Input: part model. Units: mm. Frame: model coordinates. Coordinates: 2 decimals unless noted, no trailing zeros. Write each loop counter-clockwise with the first axis right and the second up, starting at its lowest first coordinate (ties: lowest second). Pieces come first, ordered by that corner, then holes. Notation, with made-up numbers: (41, 85) - (45, 85) arc R4 cw to (45, 89) - close; hole circle Ø5 at (-20.5, 73.5). An arc over 180 degrees is marked (long way). Use CSV: the item, a comma, the result in double quotes.
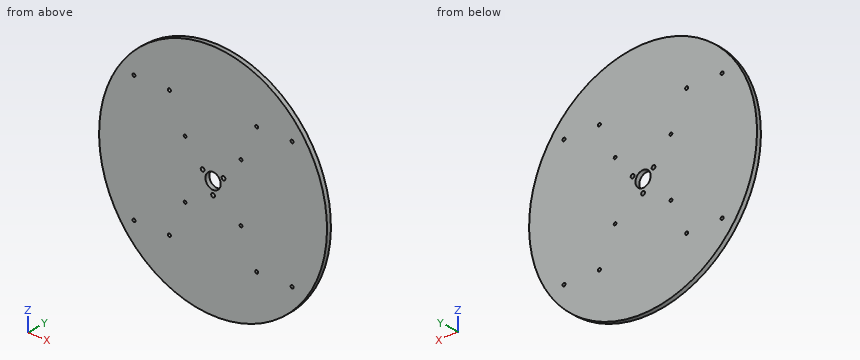
```python
from build123d import *

# Parameters (mm, degrees)
SKETCH1_R           = 165.1
BOSS_EXTRUDE1_DEPTH = 6.35
SKETCH2_R           = 11
SKETCH2_R_2         = 1.984375
SKETCH2_R_3         = 2.7
CUT_EXTRUDE1_DEPTH  = 234.572991803
SKETCH3_R           = 2.1828125
CUT_EXTRUDE2_DEPTH  = 234.572991803


with BuildPart() as part:
    # Sketch1 → Boss-Extrude1 (new body)
    with BuildSketch(Plane(origin=(0, 0, 0), x_dir=(1, 0, 0), z_dir=(0, 1, 0))):
        with Locations(Location((0, 0, 0), (0, 0, 270))):
            Circle(SKETCH1_R)
    extrude(amount=BOSS_EXTRUDE1_DEPTH)

    # Sketch2 → Cut-Extrude1 (cut, through all)
    with BuildSketch(Plane(origin=(0, 6.35, 0), x_dir=(1, 0, 0), z_dir=(0, 1, 0))):
        with Locations(Location((0, 0, 0), (0, 0, 270))):
            Circle(SKETCH2_R)
        with Locations(Location((-40.4876, 40.4876, 0), (0, 0, 270))):
            Circle(SKETCH2_R_2)
        with Locations(Location((-40.4876, -40.4876, 0), (0, 0, 270))):
            Circle(SKETCH2_R_2)
        with Locations(Location((40.4876, -40.4876, 0), (0, 0, 270))):
            Circle(SKETCH2_R_2)
        with Locations(Location((40.4876, 40.4876, 0), (0, 0, 270))):
            Circle(SKETCH2_R_2)
        with Locations(Location((0, 17.5, 0), (0, 0, 270))):
            Circle(SKETCH2_R_3)
        with Locations(Location((-15.155444566, -8.75, 0), (0, 0, 270))):
            Circle(SKETCH2_R_3)
        with Locations(Location((15.155444566, -8.75, 0), (0, 0, 270))):
            Circle(SKETCH2_R_3)
    extrude(amount=-CUT_EXTRUDE1_DEPTH, mode=Mode.SUBTRACT)

    # Sketch3 → Cut-Extrude2 (cut, through all)
    with BuildSketch(Plane(origin=(0, 6.35, 0), x_dir=(1, 0, 0), z_dir=(0, 1, 0))):
        with Locations(Location((-114.5413, 88.9, 0), (0, 0, 270))):
            Circle(SKETCH3_R)
        with Locations(Location((-63.2587, 88.9, 0), (0, 0, 270))):
            Circle(SKETCH3_R)
        with Locations(Location((63.2587, 88.9, 0), (0, 0, 270))):
            Circle(SKETCH3_R)
        with Locations(Location((114.5413, 88.9, 0), (0, 0, 270))):
            Circle(SKETCH3_R)
        with Locations(Location((114.5413, -88.9, 0), (0, 0, 270))):
            Circle(SKETCH3_R)
        with Locations(Location((63.2587, -88.9, 0), (0, 0, 270))):
            Circle(SKETCH3_R)
        with Locations(Location((-63.2587, -88.9, 0), (0, 0, 270))):
            Circle(SKETCH3_R)
        with Locations(Location((-114.5413, -88.9, 0), (0, 0, 270))):
            Circle(SKETCH3_R)
    extrude(amount=-CUT_EXTRUDE2_DEPTH, mode=Mode.SUBTRACT)


solid = part.part
```
(1) Cut plane B-B on y = 4.5. State how many separate pieces and enclosed holes the cut face has, and give its area (3 significant figures).
Check values:
separate pieces,"1"
enclosed holes,"16"
area,"85,000 mm^2"
(2) Cut plane A-A on z = 1. Return loops of the section in (x, y).
Check values:
outline,"(-165.1, 0) - (-10.95, 0) - (-10.95, 6.35) - (-165.1, 6.35) - close; (10.95, 0) - (165.1, 0) - (165.1, 6.35) - (10.95, 6.35) - close"
(3) Cut plane D-D on z = -105.5. Return loops of the section in (x, y), and give its area (3 significant figures).
Check values:
outline,"(-127, 0) - (127, 0) - (127, 6.35) - (-127, 6.35) - close"
area,"1,610 mm^2"
(4) Ray query, probe 1 along X at (y, z) = (3.75, -88.9); probe 2 along Z at (x, y) = (64, 5.5); probe 3 along Z at (x, y) = (-61.5, 4.5). Return the intervals inside material, ascending. Write a range as from..to.
Check values:
probe 1,"-139.12..-116.72, -112.36..-65.44, -61.08..61.08, 65.44..112.36, 116.72..139.12"
probe 2,"-152.19..-90.95, -86.85..86.85, 90.95..152.19"
probe 3,"-153.22..-90.19, -87.61..87.61, 90.19..153.22"
(5) Pin query (flat end, axial travel): pin 1 Ø2.5 at (x, z) = (-114.54, -88.9) entering from +Y; pin 2 Ø3 at (y, z) = (3.5, -78) entering from -X; pin 3 Ø5.5 at (x, z) = (114.54, 88.9) entering from +Y; pin 4 Ø1 at (y, z) = (5.5, -70.5) entering from -X. Return the tip coordinate at first contact, or that it passes through.
Check values:
pin 1,"through"
pin 2,"x = -146.31"
pin 3,"y = 6.35"
pin 4,"x = -149.53"
(6) Cut plane C-C on x = -49. Return loops of the section in (y, z).
Check values:
outline,"(0, -157.66) - (6.35, -157.66) - (6.35, 157.66) - (0, 157.66) - close"
